Job drawing, mm, ordinate dimensions from the low corner. One solid piece. A direction names the side the tool comes from. Round coordinates to 2 decimals unless told otherwise and drop trailing zeros. Order: outer loops, then holes, each group sorted by start corner. A loop starts at its lowest first (then second) coordinate and runs counter-clockwise, first axis right, second up. Notation, with made-up numbers: (-14.75, 74) -> (-0.75, 74) arc R23 cw to (-0.75, 92) -> close; hole circle Ø10 at (73, 22.5). An arc over 180 degrees is marked (long way). Answer as a JSON object with one key per item and string values. Group by question number.
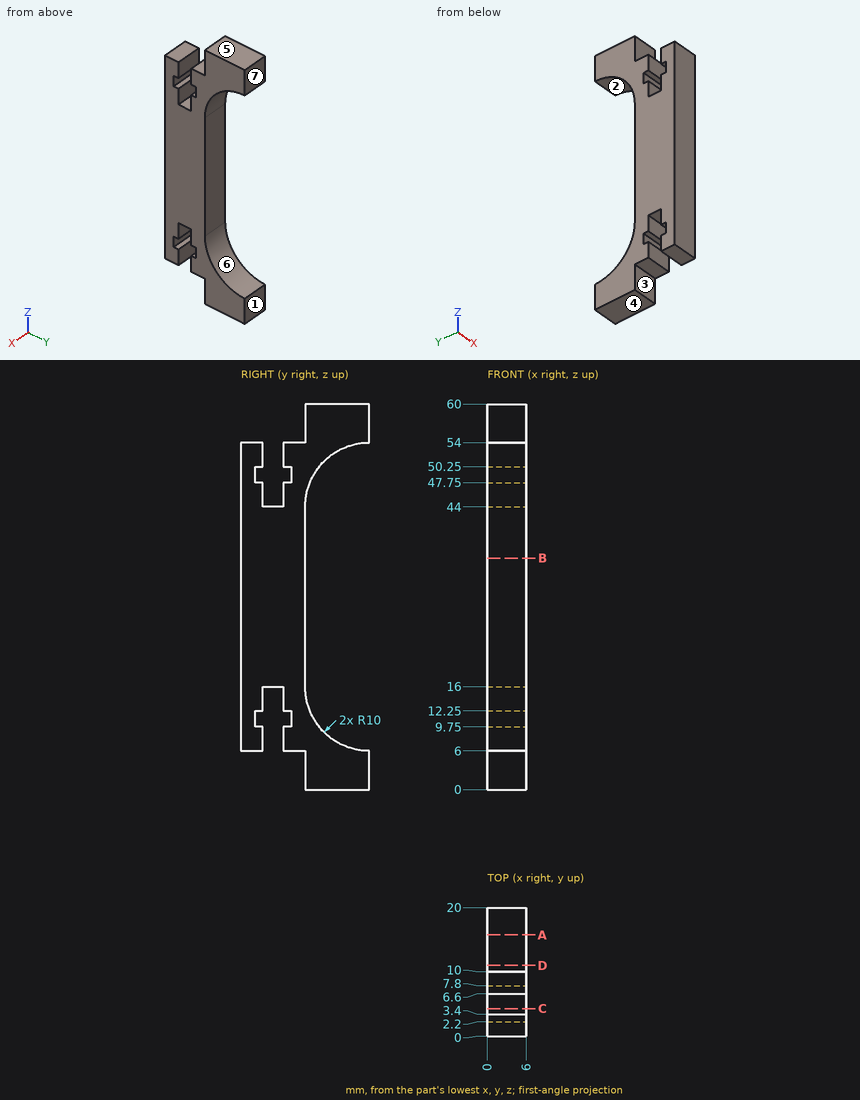
Q1. Band-saw the part on C-C (y = 4.25). List the corners of the cut face in (x, z).
Q2. Band-saw the part on B-B (z = 36). List the corners of the cut face in (x, y).
Q3. Wall check: line 1 (Z direction, x = 0.3, y = 7.75); line 2 (Z direction, x = 4.7, y = 8.5); line 3 (Y direction, x = 2.3, z = 36). Give the ranges that are in metal, low to high. Write a range as [from, to].
Q4. Two-plate mould, pull along Z, no slides. Class the marked faces 4, 5, 6 and 7: +Z half, -Z half, draft (parallel to the pull), parting line (faces both ways), or undercut.
Q5. Drop flat-ended pins along their axis: pin 1 Ø3 at (x, z) = (4, 8.5) entering from +Y; pin 2 Ø0.6 at (x, y) = (3.5, 7.5) entering from +Z; pin 3 Ø1.6 at (x, y) = (3, 5.5) entering from +Z; pin 4 Ø1 at (y, z) = (11.5, 47.5) entering from +X. Give the stop position or say it passes through.
Q6. Band-saw the part on D-D (y = 11). List the corners of the cut face in (x, z), plus the area to 3 significant figures.
Q7. Band-saw the part on A-A (y = 15.75). List the corners of the cut face in (x, z).
Q8. Which spindle directions (+Z, -Z, +X, -X, +Y, -Y) get a long thin tool onto all of the face, cutting with end or side? Do the marked faces 1, 2 and 3. Say none if no direction does.
Completed:
{
 "1": {"outline": "(0, 16) -> (6, 16) -> (6, 44) -> (0, 44) -> close"},
 "2": {"outline": "(0, 0) -> (6, 0) -> (6, 10) -> (0, 10) -> close"},
 "3": {"line 1": "[6, 9.75], [12.25, 47.75], [50.25, 54]", "line 2": "[6, 54]", "line 3": "[0, 10]"},
 "4": {"face 4": "-Z half", "face 5": "+Z half", "face 6": "undercut", "face 7": "draft"},
 "5": {"pin 1": "y = 15.64", "pin 2": "z = 54", "pin 3": "z = 44", "pin 4": "through"},
 "6": {"outline": "(0, 0) -> (6, 0) -> (6, 11.64) -> (0, 11.64) -> close; (0, 48.36) -> (6, 48.36) -> (6, 60) -> (0, 60) -> close", "area": "140 mm2"},
 "7": {"outline": "(0, 0) -> (6, 0) -> (6, 6.95) -> (0, 6.95) -> close; (0, 53.05) -> (6, 53.05) -> (6, 60) -> (0, 60) -> close"},
 "8": {"face 1": "+Z, -Z, +X, -X, +Y", "face 2": "+X, -X, +Y", "face 3": "-Z, +X, -X, -Y"}
}
